```python
from build123d import *

# Parameters (mm, degrees)
BOSS_EXTRU_1_DEPTH = 100
CONG_2_R           = 1
CONGES_BASE_R      = 20
CONG_4_R           = 1
CONG_5_R           = 5


with BuildPart() as part:
    # Esquisse1 → Boss.-Extru.1 (new body)
    with BuildSketch(Plane.XY):
        Polygon((-11.5, 2.4), (11.5, 2.4), (11.5, 80), (13.9, 66.111581736), (13.9, 2.4), (29.296036477, 2.4), (32.866170168, 8.646815683), (36.954561628, 24.631379819), (40, 7.007912357), (40, 0), (-40, 0), (-40, 7.007912357), (-36.954561628, 24.631379819), (-32.866170168, 8.646815683), (-29.296036477, 2.4), (-13.9, 2.4), (-13.9, 66.111581736), (-11.5, 80), (-11.5, 60), (-9, 60), (-9, 50), (-11.5, 50), align=None)
    extrude(amount=BOSS_EXTRU_1_DEPTH)

    # Congé2
    cong_2_edges = [part.edges().sort_by_distance(p)[0] for p in [
        (-11.5, 60, 50),
        (-9, 60, 50),
        (-9, 50, 50),
        (-11.5, 50, 50),
    ]]
    fillet(cong_2_edges, radius=CONG_2_R)

    # Conges_base
    # the kernel refuses this fillet: 20 mm, written as the material it adds along each edge
    with BuildSketch(Plane(origin=(13.9, 2.4, 0), x_dir=(0, 1, 0), z_dir=(0, 0, 1))) as conges_base_piece_1:
        with BuildLine():
            CenterArc((19.462875427, -20), CONGES_BASE_R, 90, 76.691260518)
            Line((0, -15.396036477), (-0.389257509, -15.303957207))
            ThreePointArc((-0.389257509, -15.303957207), (-0.4, -7.698018239), (-0.4, 0))
            Line((-0.4, 0), (0, 0.4))
            Line((0, 0.4), (19.462875427, 0.4))
            Line((19.462875427, 0.4), (19.462875427, 0))
        make_face()
    extrude(amount=100)
    with BuildSketch(Plane(origin=(-13.9, 2.4, 0), x_dir=(0, 1, 0), z_dir=(0, 0, 1))) as conges_base_piece_2:
        with BuildLine():
            CenterArc((19.462875427, 20), CONGES_BASE_R, 193.308739482, 76.691260518)
            Line((0, 15.396036477), (-0.389257509, 15.303957207))
            ThreePointArc((-0.389257509, 15.303957207), (-0.4, 7.698018239), (-0.4, 0))
            Line((-0.4, 0), (0, -0.4))
            Line((0, -0.4), (19.462875427, -0.4))
            Line((19.462875427, -0.4), (19.462875427, 0))
        make_face()
    extrude(amount=100)

    # Congé4
    cong_4_edges = [part.edges().sort_by_distance(p)[0] for p in [
        (11.5, 80, 50),
        (36.954561628, 24.631379819, 50),
        (40, 0, 50),
        (-40, 0, 50),
        (-36.954561628, 24.631379819, 50),
        (-11.5, 80, 50),
    ]]
    fillet(cong_4_edges, radius=CONG_4_R)

    # Congé5
    cong_5_edges = [part.edges().sort_by_distance(p)[0] for p in [
        (29.296036477, 2.4, 50),
        (-29.296036477, 2.4, 50),
    ]]
    fillet(cong_5_edges, radius=CONG_5_R)


solid = part.part
```
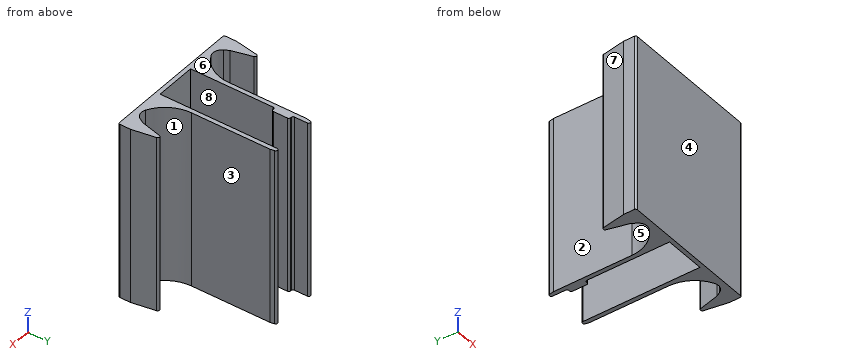
Input: part model. Units: mm. Frame: model coordinates. Face numbers are marked on the shaded views. A direction names the side the tool comes from. Round coordinates to 2 decimals unless told otherwise and drop trailing zeros. Loops run counter-clockwise (first coordinate to the right, second up) from the corner with the lowest first, then second, coordinate; pieces in that order, holes last. Notation, with made-up numbers: (17.5, 47) -> (62.5, 47) arc R10 ccw to (62.5, 66) -> close; hole circle Ø3 at (-12.5, 76). An arc over 180 degrees is marked (long way). Use one line per item in the form item = value. Start each with the question number.
Item 1: Section query B-B on y = 10.5. Return the cut outline in (x, z), then the cut area to 3 significant figures.
Item 2: Contact query for flat-ended pins moving along their axis: pin 1 Ø12 at (y, z) = (33.5, 43.5) entering from +X; pin 2 Ø1.5 at (x, z) = (-7.5, 88.5) entering from +Y; pin 3 Ø1.5 at (x, z) = (-20, 12.5) entering from +Y; pin 4 Ø8 at (x, y) = (20.5, 51.5) entering from +Z. Output: stop coordinate, or through.
Item 3: Mould query, pull axis X, two halves, no side actions, for the marked faces 5, 6, 7 and 8. Classes: pulls with the +X half, pulls with the -X half, needs draft (parallel to the pull), parting line crosses it, or undercut.
Item 4: Section query D-D on x = 8.5. Return the cut outline in (y, z), then the cut area to 3 significant figures.
Item 5: Set-up query: the marked faces 1, 2, 3 and 4. Return all of +Z, -Z, +X, -X, +Y, -Y with unobstructed straight access to the full face (end or side cutting, diameter ignored); none if empty.
Item 6: Section query A-A on y = 47.5. Return the cut outline in (x, z), then the cut area to 3 significant figures.
Item 7: Material intervals for L1, parallel to X at y = 24, z = 27.5; L2, parallel to Y at x = -10, z = 10; L3, parallel to X at y = 18, z = 84, sorted ascending. Write a range as from..to.
Ans:
q1.outline = (-39.4, 0) -> (-33.34, 0) -> (-33.34, 100) -> (-39.4, 100) -> close; (-17.44, 0) -> (-11.5, 0) -> (-11.5, 100) -> (-17.44, 100) -> close; (11.5, 0) -> (17.44, 0) -> (17.44, 100) -> (11.5, 100) -> close; (33.34, 0) -> (39.4, 0) -> (39.4, 100) -> (33.34, 100) -> close
q1.area = 2,400 mm^2
q2.pin_1 = 13.9
q2.pin_2 = 2.4
q2.pin_3 = 8.25
q2.pin_4 = through
q3.face_5 = undercut
q3.face_6 = needs draft
q3.face_7 = pulls with the -X half
q3.face_8 = undercut
q4.outline = (0, 0) -> (2.4, 0) -> (2.4, 100) -> (0, 100) -> close
q4.area = 240 mm^2
q5.face_1 = +Z, -Z, +Y
q5.face_2 = +Z, -Z, -X, +Y
q5.face_3 = +Z, -Z, +X, +Y
q5.face_4 = +Z, -Z, +X, -X, -Y
q6.outline = (-13.9, 0) -> (-11.5, 0) -> (-11.5, 100) -> (-13.9, 100) -> close; (11.5, 0) -> (13.9, 0) -> (13.9, 100) -> (11.5, 100) -> close
q6.area = 480 mm^2
q7.L1 = -13.9..-11.5, 11.5..13.9
q7.L2 = 0..2.4, 50..60
q7.L3 = -38.1..-35.26, -14.28..-11.5, 11.5..14.28, 35.26..38.1
